from build123d import *

# Parameters (mm, degrees)
SKETCH1_W           = 44.05
SKETCH1_H           = 31.35
SKETCH1_R           = 1.4
BOSS_EXTRUDE1_DEPTH = 20
SKETCH2_W           = 44.05
SKETCH2_H           = 31.35
BOSS_EXTRUDE2_DEPTH = 1.7
SKETCH3_W           = 2.9
SKETCH3_H           = 15.7
SKETCH3_W_2         = 4.9
SKETCH3_H_2         = 14
SKETCH3_H_3         = 5.5
BOSS_EXTRUDE3_DEPTH = 14.15
SKETCH4_W           = 4.9
SKETCH4_H           = 14
SKETCH4_W_2         = 2.5
SKETCH4_H_2         = 5.1
SKETCH4_H_3         = 15.3
BOSS_EXTRUDE4_DEPTH = 2.85
SKETCH5_W           = 1.4
SKETCH5_H           = 5
SKETCH5_W_2         = 1.2
SKETCH5_H_2         = 5.1
CUT_EXTRUDE1_DEPTH  = 2.85
CUT_EXTRUDE2_REACH  = 23.7


with BuildPart() as part:
    # Sketch1 → Boss-Extrude1 (new body)
    with BuildSketch(Plane.XY):
        Rectangle(SKETCH1_W, SKETCH1_H)
        with Locations((-17.7875, -11.45)):
            Circle(SKETCH1_R, mode=Mode.SUBTRACT)
        with Locations((17.7875, -11.45)):
            Circle(SKETCH1_R, mode=Mode.SUBTRACT)
        with BuildLine():
            Line((-17.7875, -8.45), (-20.525, -8.45))
            Line((-20.525, -8.45), (-20.525, 8.45))
            Line((-20.525, 8.45), (-17.7875, 8.45))
            ThreePointArc((-17.7875, 8.45), (-15.666179656, 9.328679656), (-14.7875, 11.45))
            Line((-14.7875, 11.45), (-14.7875, 14.175))
            Line((-14.7875, 14.175), (14.7875, 14.175))
            Line((14.7875, 14.175), (14.7875, 11.45))
            ThreePointArc((14.7875, 11.45), (15.666179656, 9.328679656), (17.7875, 8.45))
            Line((17.7875, 8.45), (20.525, 8.45))
            Line((20.525, 8.45), (20.525, -8.45))
            Line((20.525, -8.45), (17.7875, -8.45))
            ThreePointArc((17.7875, -8.45), (15.666179656, -9.328679656), (14.7875, -11.45))
            Line((14.7875, -11.45), (14.7875, -14.175))
            Line((14.7875, -14.175), (-14.7875, -14.175))
            Line((-14.7875, -14.175), (-14.7875, -11.45))
            ThreePointArc((-14.7875, -11.45), (-15.666179656, -9.328679656), (-17.7875, -8.45))
        make_face(mode=Mode.SUBTRACT)
        with Locations((-17.7875, 11.45)):
            Circle(SKETCH1_R, mode=Mode.SUBTRACT)
        with Locations((17.7875, 11.45)):
            Circle(SKETCH1_R, mode=Mode.SUBTRACT)
    extrude(amount=BOSS_EXTRUDE1_DEPTH)

    # Sketch2 → Boss-Extrude2 (add)
    with BuildSketch(Plane(origin=(0, 0, 0), x_dir=(-1, 0, 0), z_dir=(0, 0, -1))):
        Rectangle(SKETCH2_W, SKETCH2_H)
        Polygon((-20.525, 8.45), (-20.525, 14.175), (-14.7875, 14.175), (-2, 14.175), (-2, 14.925), (2, 14.925), (2, 14.175), (14.7875, 14.175), (20.525, 14.175), (20.525, 8.45), (20.525, 2), (21.275, 2), (21.275, -2), (20.525, -2), (20.525, -8.45), (20.525, -14.175), (14.7875, -14.175), (2, -14.175), (2, -14.925), (-2, -14.925), (-2, -14.175), (-14.7875, -14.175), (-20.525, -14.175), (-20.525, -8.45), (-20.525, -2), (-21.275, -2), (-21.275, 2), (-20.525, 2), align=None, mode=Mode.SUBTRACT)
    extrude(amount=BOSS_EXTRUDE2_DEPTH)

    # Sketch3 → Boss-Extrude3 (add)
    with BuildSketch(Plane(origin=(0, 0, 3), x_dir=(-1, 0, 0), z_dir=(0, 0, -1))):
        with BuildLine():
            ThreePointArc((16.225, -8.889024844), (16.975996909, -8.561840944), (17.7875, -8.45))
            Line((17.7875, -8.45), (20.525, -8.45))
            Line((20.525, -8.45), (20.525, 8.45))
            Line((20.525, 8.45), (17.7875, 8.45))
            ThreePointArc((17.7875, 8.45), (16.975996909, 8.561840944), (16.225, 8.889024844))
            Line((16.225, 8.889024844), (16.225, -8.889024844))
        make_face()
        with Locations((18.875, 0)):
            Rectangle(SKETCH3_W, SKETCH3_H, mode=Mode.SUBTRACT)
        with Locations((-8.875, -7.175)):
            Rectangle(SKETCH3_W_2, SKETCH3_H_2)
        with Locations((-8.875, -3.925)):
            Rectangle(SKETCH3_W, SKETCH3_H_3, mode=Mode.SUBTRACT)
    extrude(amount=-BOSS_EXTRUDE3_DEPTH)

    # Sketch4 → Boss-Extrude4 (add)
    with BuildSketch(Plane.XY.offset(17.15)):
        with Locations((8.875, -7.175)):
            Rectangle(SKETCH4_W, SKETCH4_H)
        with Locations((8.875, -3.925)):
            Rectangle(SKETCH4_W_2, SKETCH4_H_2, mode=Mode.SUBTRACT)
        with BuildLine():
            Line((-20.525, -8.45), (-17.7875, -8.45))
            ThreePointArc((-17.7875, -8.45), (-16.975996909, -8.561840944), (-16.225, -8.889024844))
            Line((-16.225, -8.889024844), (-16.225, 8.889024844))
            ThreePointArc((-16.225, 8.889024844), (-16.975996909, 8.561840944), (-17.7875, 8.45))
            Line((-17.7875, 8.45), (-20.525, 8.45))
            Line((-20.525, 8.45), (-20.525, -8.45))
        make_face()
        with Locations((-18.875, 0)):
            Rectangle(SKETCH4_W_2, SKETCH4_H_3, mode=Mode.SUBTRACT)
    extrude(amount=BOSS_EXTRUDE4_DEPTH)

    # Sketch5 → Cut-Extrude1 (cut)
    with BuildSketch(Plane.XY.offset(20)):
        with Locations((-16.925, 0)):
            Rectangle(SKETCH5_W, SKETCH5_H)
        with Locations((7.025, -3.925)):
            Rectangle(SKETCH5_W_2, SKETCH5_H_2)
    extrude(amount=-CUT_EXTRUDE1_DEPTH, mode=Mode.SUBTRACT)

    # Sketch6 → Cut-Extrude2 (cut, up to next)
    with BuildSketch(Plane(origin=(0, 0, -1.7), x_dir=(-1, 0, 0), z_dir=(0, 0, -1)), mode=Mode.PRIVATE) as cut_extrude2_sk1:
        with BuildLine():
            Line((-18.112740296, 15.675), (-22.025, 15.675))
            Line((-22.025, 15.675), (-22.025, 11.45))
            ThreePointArc((-22.025, 11.45), (-20.896729165, 14.329079757), (-18.112740296, 15.675))
        make_face()
    cut_extrude2_tool1 = extrude(cut_extrude2_sk1.sketch, amount=-CUT_EXTRUDE2_REACH, mode=Mode.PRIVATE) & part.part
    add(cut_extrude2_tool1.solids().sort_by_distance((21.092545, 14.728552, -1.7))[0], mode=Mode.SUBTRACT)
    # Sketch6 → Cut-Extrude2 (cut, up to next)
    with BuildSketch(Plane(origin=(0, 0, -1.7), x_dir=(-1, 0, 0), z_dir=(0, 0, -1)), mode=Mode.PRIVATE) as cut_extrude2_sk2:
        with BuildLine():
            Line((22.025, 15.675), (18.112740296, 15.675))
            ThreePointArc((18.112740296, 15.675), (20.896729165, 14.329079757), (22.025, 11.45))
            Line((22.025, 11.45), (22.025, 15.675))
        make_face()
    cut_extrude2_tool2 = extrude(cut_extrude2_sk2.sketch, amount=-CUT_EXTRUDE2_REACH, mode=Mode.PRIVATE) & part.part
    add(cut_extrude2_tool2.solids().sort_by_distance((-21.092545, 14.728552, -1.7))[0], mode=Mode.SUBTRACT)
    # Sketch6 → Cut-Extrude2 (cut, up to next)
    with BuildSketch(Plane(origin=(0, 0, -1.7), x_dir=(-1, 0, 0), z_dir=(0, 0, -1)), mode=Mode.PRIVATE) as cut_extrude2_sk3:
        with BuildLine():
            Line((22.025, -15.675), (22.025, -11.45))
            ThreePointArc((22.025, -11.45), (20.896729165, -14.329079757), (18.112740296, -15.675))
            Line((18.112740296, -15.675), (22.025, -15.675))
        make_face()
    cut_extrude2_tool3 = extrude(cut_extrude2_sk3.sketch, amount=-CUT_EXTRUDE2_REACH, mode=Mode.PRIVATE) & part.part
    add(cut_extrude2_tool3.solids().sort_by_distance((-21.092545, -14.728552, -1.7))[0], mode=Mode.SUBTRACT)
    # Sketch6 → Cut-Extrude2 (cut, up to next)
    with BuildSketch(Plane(origin=(0, 0, -1.7), x_dir=(-1, 0, 0), z_dir=(0, 0, -1)), mode=Mode.PRIVATE) as cut_extrude2_sk4:
        with BuildLine():
            ThreePointArc((-18.112740296, -15.675), (-20.896729167, -14.329079755), (-22.025, -11.449999993))
            Line((-22.025, -11.449999993), (-22.025, -15.675))
            Line((-22.025, -15.675), (-18.112740296, -15.675))
        make_face()
    cut_extrude2_tool4 = extrude(cut_extrude2_sk4.sketch, amount=-CUT_EXTRUDE2_REACH, mode=Mode.PRIVATE) & part.part
    add(cut_extrude2_tool4.solids().sort_by_distance((21.092545, -14.728552, -1.7))[0], mode=Mode.SUBTRACT)


solid = part.part
Here's how the part is built. I have some questions about the finished solid (model axes, mm). A direction names the side the tool comes from. Round coordinates to 2 decimals unless told otherwise and drop trailing zeros. Loops run counter-clockwise (first coordinate to the right, second up) from the corner with the lowest first, then second, coordinate; pieces in that order, holes last. Notation, with made-up numbers: (39, 36) -> (60, 36) arc R17 ccw to (60, 61) -> close; hole circle Ø4 at (3, 80). An arc over 180 degrees is marked (long way). Write each question's results on one line, items separated by ' | '.
(1) For faces 1 (the face through (21.275, 0, -1)), 2 (the face through (6.425, -7, 11)), which set-ups out of +Z, -Z, +X, -X, +Y, -Y let a thin tool reach every point of the face, with its end or its side?
Worked answers:
face 1: -Z | face 2: +Z, -Z
(2) If we section it at B-B, the plane y = 5.5: List the corners of the cut face in (x, z) for me (3 decimals), then the cut area to 3 significant figures.
Worked answers:
outline: (-22.025, -1.7) -> (-20.525, -1.7) -> (-20.525, 3) -> (-20.325, 3) -> (-20.325, 17.15) -> (-20.125, 17.15) -> (-20.125, 20) -> (-22.025, 20) -> close; (-17.625, 17.15) -> (-17.425, 17.15) -> (-17.425, 3) -> (-16.225, 3) -> (-16.225, 20) -> (-17.625, 20) -> close; (20.525, -1.7) -> (22.025, -1.7) -> (22.025, 20) -> (20.525, 20) -> close | area: 90.0 mm2
(3) If I drill on L1, parallel to Y at x = 10, z = 17.5 (3 decimals); L2, parallel to X at y = 1.5, z = 10.25 (3 decimals); L3, parallel to Y at x = 8, z = 8 (3 decimals), over which ranges is the centre line in solid material (lowest first)?
Worked answers:
L1: -15.675 to -6.475, -1.375 to -0.175, 14.175 to 15.675 | L2: -22.025 to -20.325, -17.425 to -16.225, 20.525 to 22.025 | L3: -15.675 to -6.675, -1.175 to -0.175, 14.175 to 15.675
(4) For P1, Ø0.9, axis at x = 9, y = -5, coming from the -Z side; P2, Ø3, axis at x = 17.79, y = -11.45, coming from the -Z side; P3, Ø1, axis at x = -16.5, y = -0.5, coming from the +Z side, each with a flat end and sliding along its axis, tell me the tip position at first contact or that it passes through.
Worked answers:
P1: through | P2: z = 0 | P3: z = 17.15
(5) If we section it at A-A, the plane x = -3: List the corners of the cut face in (y, z) for me (3 decimals), then the cut area to 3 significant figures.
Worked answers:
outline: (-15.675, -1.7) -> (-14.175, -1.7) -> (-14.175, 20) -> (-15.675, 20) -> close; (14.175, -1.7) -> (15.675, -1.7) -> (15.675, 20) -> (14.175, 20) -> close | area: 65.1 mm2
(6) We'd pull the mould along X, two halves only. Please class faces 3 (the face through (-14.788, -13, 10)), 4 (the face through (22.025, 0, 9)), 5 (the face through (0.1, 15.2, -1.7)): released by +X, released by -X, zero draft, split by the parting line, or undercut.
Worked answers:
face 3: undercut | face 4: released by +X | face 5: zero draft
(7) If we section it at C-C, the plane x = 9.5: List the corners of the cut face in (y, z) for me (3 decimals), then the cut area to 3 significant figures.
Worked answers:
outline: (-15.675, -1.7) -> (-14.175, -1.7) -> (-14.175, 3) -> (-6.675, 3) -> (-6.675, 17.15) -> (-6.475, 17.15) -> (-6.475, 20) -> (-15.675, 20) -> close; (-1.375, 17.15) -> (-1.175, 17.15) -> (-1.175, 3) -> (-0.175, 3) -> (-0.175, 20) -> (-1.375, 20) -> close; (14.175, -1.7) -> (15.675, -1.7) -> (15.675, 20) -> (14.175, 20) -> close | area: 211 mm2
(8) If we section it at D-D, the plane z = 2.5: Give the number of separate pieces and of enclosed holes in the cut face, then the cut area to 3 significant figures.
Worked answers:
separate pieces: 1 | enclosed holes: 5 | area: 301 mm2
